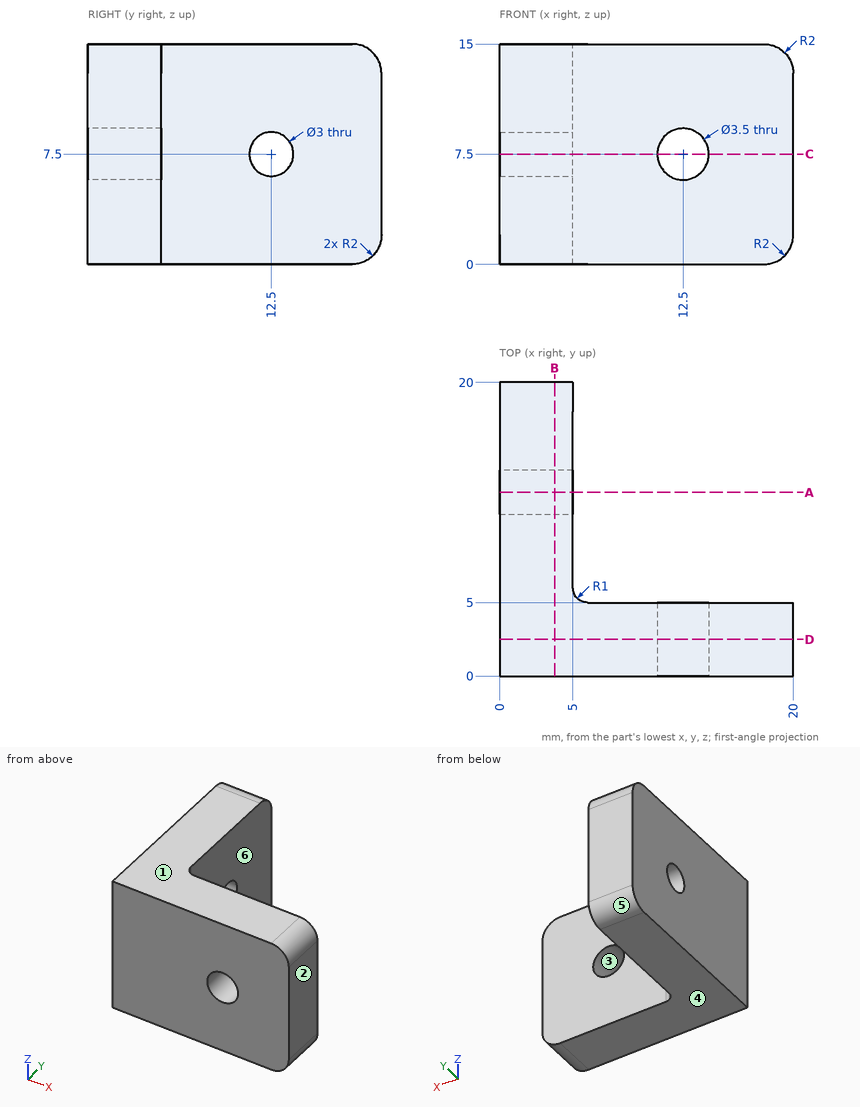
Geometry: see drawing. Coordinates: mm, zero at the bounding-box minimum. A direction names the side the tool comes from. Give positions to 0.01 mm unless a question says otherwise; leave off trailing zeros. Loops run counter-clockwise (first coordinate to the right, second up) from the corner with the lowest first, then second, coordinate; pieces in that order, holes last. Notation, with made-up numbers: (13, 49) -> (60, 49) arc R20 ccw to (60, 87) -> close; hole circle Ø5 at (35.5, -16.5). An arc over 180 degrees is marked (long way). Answer as a JSON object with one key per item and string values. Group by question number.
Item 1: Pin query (flat end, axial travel): P1, Ø4, axis at y = 12.5, z = 7.5, coming from the +X side; P2, Ø4, axis at x = 12.5, z = 10, coming from the +Y side. Return the tip coordinate at first contact, or that it passes through.
Item 2: Cut plane C-C, the plane z = 7.5. Return the cut outline in (x, y), and give its area (3 significant figures).
Item 3: Cut plane A-A, the plane y = 12.5. Return the cut outline in (x, z).
Item 4: Line query: probe 1 along Z at (x, y) = (1.7, 12.5); probe 2 along Z at (x, y) = (12.5, 3.4); probe 3 along Y at (x, z) = (9, 4). Output: solid intervals per line, ascending.
Item 5: Reachability of the marked faces 5 and 6 from +Z, -Z, +X, -X, +Y, -Y: full face, straight path, thin tool, end or side. Return the list, or none.
Item 6: Pull-direction query (Z, two-part tool) for the marked faces 1, 2, 3 and 4; classes: released by +Z, released by -Z, zero draft, split by the parting line, or undercut.
Item 7: Cut plane B-B, the plane x = 3.75. Return the cut outline in (y, z).
Item 8: Cut plane D-D, the plane y = 2.5. Return the cut outline in (x, z), and give its area (3 significant figures).
Checks:
{
 "1": {"P1": "stops at x = 5", "P2": "stops at y = 5"},
 "2": {"outline": "(0, 0) -> (10.75, 0) -> (10.75, 5) -> (6, 5) arc R1 cw to (5, 6) -> (5, 11) -> (0, 11) -> close; (0, 14) -> (5, 14) -> (5, 20) -> (0, 20) -> close; (14.25, 0) -> (20, 0) -> (20, 5) -> (14.25, 5) -> close", "area": "143 mm²"},
 "3": {"outline": "(0, 0) -> (5, 0) -> (5, 6) -> (0, 6) -> close; (0, 9) -> (5, 9) -> (5, 15) -> (0, 15) -> close"},
 "4": {"probe 1": "z = 0 to 6, 9 to 15", "probe 2": "z = 0 to 5.75, 9.25 to 15", "probe 3": "y = 0 to 5"},
 "5": {"face 5": "-Z, +X, -X, +Y", "face 6": "+Z, -Z, +X, +Y"},
 "6": {"face 1": "released by +Z", "face 2": "zero draft", "face 3": "undercut", "face 4": "released by -Z"},
 "7": {"outline": "(0, 0) -> (18, 0) arc R2 ccw to (20, 2) -> (20, 13) arc R2 ccw to (18, 15) -> (0, 15) -> close; hole circle Ø3 at (12.5, 7.5)"},
 "8": {"outline": "(0, 0) -> (18, 0) arc R2 ccw to (20, 2) -> (20, 13) arc R2 ccw to (18, 15) -> (0, 15) -> close; hole circle Ø3.5 at (12.5, 7.5)", "area": "289 mm²"}
}
